Autodesk Inventor part; units mm, degrees
ref_plane "YZ Plane" through (0, 0, 0) normal (1, 0, 0) x (0, 1, 0)
ref_plane "XZ Plane" through (0, 0, 0) normal (0, 1, 0) x (-1, 0, 0)
ref_plane "XY Plane" through (0, 0, 0) normal (0, 0, 1) x (1, 0, 0)
sketch "スケッチ1" plane through (0, 0, 0) normal (0, 0, 1) x (1, 0, 0)
  line L0 (0, 0) -> (100, 0)
  line L1 (100, 0) -> (100, 300)
  line L2 (100, 300) -> (0, 300)
  line L3 (0, 300) -> (0, 0)
  line L4 (0, 218) -> (40, 218)
  line L5 (40, 218) -> (40, 82)
  line L6 (40, 82) -> (0, 82)
  line L7 (0, 82) -> (0, 218)
  point P0 (0, 150)
  point P1 (40, 150)
  point P2 (0, 82)
  dimension "d0" = 136
  dimension "d1" = 300
  dimension "d2" = 100
  dimension "d3" = 40
  dimension "d4" = 0
extrude "押し出し1" add sketch "スケッチ1" along normal blind 10 contours L3 L6 L5 L4 L2 L1 L0
properties part number "base"
The model under review builds one solid part; all positions refer to its coordinate system, in mm. A direction names the side the tool comes from. Coordinates: 2 decimals unless noted, no trailing zeros. Write each loop counter-clockwise with the first axis right and the second up, starting at its lowest first coordinate (ties: lowest second). Pieces come first, ordered by that corner, then holes. Notation, with made-up numbers: (0, 77.5) - (30, 77.5) arc R19 ccw to (30, 110.5) - close; hole circle Ø2 at (18, -15.5). An arc over 180 degrees is marked (long way). Answer as a JSON object with one key per item and string values. Group by question number.
1. Add section B-B (z = 4). Give the boundary of the cut face in (x, y), plus the area to 3 significant figures.
2. Machinability: for faces 4 (the face through (20, 82, 5)), 5 (the face through (100, 148, 5)), which of the approach directions +Z, -Z, +X, -X, +Y, -Y give a long, thin tool a straight path to every point of the face, cutting with its end or side? Answer none if there is none.
3. To check wall thickness, follow probe 1 along Y at (x, z) = (33.5, 6); probe 2 along X at (y, z) = (160.5, 5.25). State the ranges of each line that lie inside material, in increasing order.
4. Add section C-C (y = 165). Give the boundary of the cut face in (x, z), plus the area to 3 significant figures.
5. Clearance check with a flat-ended pin moving along its axis: pin 1 Ø5 at (y, z) = (169, 3.5) entering from -X. State where the tip first meets the part, or that it passes through.
6. Mouldability with a two-part tool opening along Y and no side actions: class faces 1 (the face through (60, 152, 10)), 2 (the face through (40, 151, 5)), 3 (the face through (49, 0, 5)) as pulls with the +Y half, pulls with the -Y half, needs draft (parallel to the pull), parting line crosses it, or undercut.
7. Add section A-A (x = 20.5). Give the boundary of the cut face in (y, z).
Findings:
{
 "1": {"outline": "(0, 0) - (100, 0) - (100, 300) - (0, 300) - (0, 218) - (40, 218) - (40, 82) - (0, 82) - close", "area": "24,600 mm²"},
 "2": {"face 4": "+Z, -Z, -X", "face 5": "+Z, -Z, +X, +Y, -Y"},
 "3": {"probe 1": "0 to 82, 218 to 300", "probe 2": "40 to 100"},
 "4": {"outline": "(40, 0) - (100, 0) - (100, 10) - (40, 10) - close", "area": "600 mm²"},
 "5": {"pin 1": "x = 40"},
 "6": {"face 1": "needs draft", "face 2": "undercut", "face 3": "pulls with the -Y half"},
 "7": {"outline": "(0, 0) - (82, 0) - (82, 10) - (0, 10) - close; (218, 0) - (300, 0) - (300, 10) - (218, 10) - close"}
}
